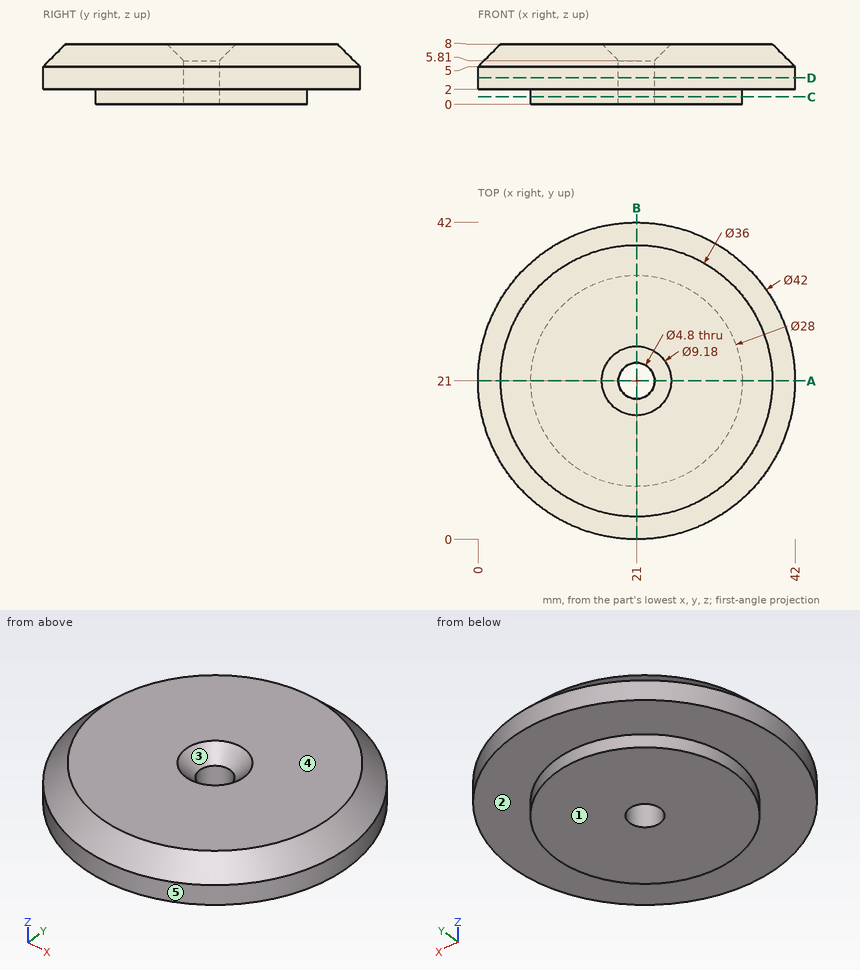
Study the drawing (mm; zero at the part's minimum x, y, z) and answer. A direction names the side the tool comes from. Coordinates: 2 decimals unless noted, no trailing zeros. Order: outer loops, then holes, each group sorted by start corner. A loop starts at its lowest first (then second) coordinate and runs counter-clockwise, first axis right, second up. Notation, with made-up numbers: (-29.5, -25) -> (-24.5, -25) arc R31 cw to (-24.5, 2) -> close; hole circle Ø3 at (-20.5, 84). An arc over 180 degrees is marked (long way). Answer in a Markdown table with one row per item. Add a question column.
Item 1: Find section D-D (z = 3.5). Write down the section's boundary in (x, y).
Item 2: Find the intervals of material crossed by L1, parallel to X at y = 21, z = 1.4; L2, parallel to X at y = 21, z = 2.8, in increasing order. Write a range as from..to.
Item 3: Find section A-A (y = 21). Write down the section's boundary in (x, z), then the cut area to 3 significant figures.
Item 4: Determine the mould class of the marked faces 3, 4 and 5 for opening direction Y: +Y half, -Y half, draft (parallel to the pull), parting line (faces both ways), or undercut.
Item 5: Which of the six approach directions +Z, -Z, +X, -X, +Y, -Y give full straight-line access (tool end or side, diameter ignored) to the marked faces 1 and 2?
Item 6: Find section C-C (z = 1). Write down the section's boundary in (x, y).
Item 7: Each of these flat-tipped pins is pushed along its axis until it touches: P1, Ø1.5, axis at x = 19, z = 3, coming from the +Y side; P2, Ø1.5, axis at y = 22, z = 1.5, coming from the +X side; P3, Ø1, axis at x = 21, y = 18, coming from the +Z side. Where does it stop, or does it pass through?
Result set:
| question | item | result |
|---|---|---|
| 1 | outline | circle Ø42 at (21, 21); hole circle Ø4.8 at (21, 21) |
| 2 | L1 | x = 7..18.6, 23.4..35 |
| 2 | L2 | x = 0..18.6, 23.4..42 |
| 3 | outline | (0, 2) -> (7, 2) -> (7, 0) -> (18.6, 0) -> (18.6, 5.81) -> (16.41, 8) -> (3, 8) -> (0, 5) -> close; (23.4, 0) -> (35, 0) -> (35, 2) -> (42, 2) -> (42, 5) -> (39, 8) -> (25.59, 8) -> (23.4, 5.81) -> close |
| 3 | area | 256 mm² |
| 4 | face 3 | undercut |
| 4 | face 4 | draft |
| 4 | face 5 | parting line |
| 5 | face 1 | -Z, +X, -X, +Y, -Y |
| 5 | face 2 | -Z |
| 6 | outline | circle Ø28 at (21, 21); hole circle Ø4.8 at (21, 21) |
| 7 | P1 | stops at y = 41.96 |
| 7 | P2 | stops at x = 42 |
| 7 | P3 | stops at z = 6.91 |
